Autodesk Inventor part; units mm, degrees
ref_plane "YZ Plane" through (0, 0, 0) normal (1, 0, 0) x (0, 1, 0)
ref_plane "XZ Plane" through (0, 0, 0) normal (0, 1, 0) x (-1, 0, 0)
ref_plane "XY Plane" through (0, 0, 0) normal (0, 0, 1) x (1, 0, 0)
sketch "Sketch1" plane through (0, 0, 0) normal (0, 1, 0) x (-1, 0, 0)
  line L0 (0, 0) -> (60, 0)
  line L1 (60, 0) -> (60, -60)
  line L2 (60, -60) -> (0, -60)
  line L3 (0, -60) -> (0, 0)
  dimension "d0" = 60
  dimension "d1" = 60
extrude "Extrusion1" add sketch "Sketch1" along normal blind 3
sketch "Sketch2" plane through (0, 3, 0) normal (0, 1, 0) x (1, 0, 0)
  line L0 (-60, 0) -> (0, 0)
  line L1 (-60, 60) -> (-60, 0)
  point P0 (-55, 5)
  dimension "d4" = 5
  dimension "d5" = 5
hole "Hole1" at (-55, 3, -5) direction (0, -1, 0) diameter 3 end through all
ref_plane "Work Plane1" through (-30, 0, -60) normal (-1, 0, 0) x (0, 0, 1)
ref_plane "Work Plane2" through (-60, 0, -30) normal (0, 0, 1) x (1, 0, 0)
mirror "Mirror1" about plane through (-30, 0, -60) normal (-1, 0, 0) of "Hole1"
mirror "Mirror2" about plane through (-60, 0, -30) normal (0, 0, 1) of "Hole1", "Mirror1"
sketch "Sketch3" plane through (0, 0, 0) normal (0, -1, 0) x (1, 0, 0)
  line L0 (-39.5, 0) -> (-34.5, 0)
  line L1 (-34.5, 0) -> (-34.5, -60)
  line L2 (-34.5, -60) -> (-39.5, -60)
  line L3 (-39.5, -60) -> (-39.5, 0)
  line L4 (0, -60) -> (-60, -60)
  line L5 (-60, 0) -> (0, 0)
  line L6 (-30, -72) -> (-30, 12)
  dimension "d13" = 5
  dimension "d14" = 4.5
extrude "Extrusion2" add sketch "Sketch3" along normal blind 10 contours L0 L1 L2 L3
sketch "Sketch4" plane through (-34.5, 0, 0) normal (1, 0, 0) x (0, 0, -1)
  line L0 (0, 0) -> (0, -10)
  line L1 (60, 0) -> (60, -10)
  line L2 (0, 0) -> (60, 0)
  line L3 (60, -10) -> (0, -10)
  point P0 (5, -7)
  point P1 (55, -7)
  dimension "d17" = 5
  dimension "d18" = 5
  dimension "d20" = 3
  dimension "d21" = 3
hole "Hole2" at (-34.5, -7, -5) at (-34.5, -7, -55) direction (-1, 0, 0) diameter 3 end through all
mirror "Mirror3" about plane through (-30, 0, -60) normal (-1, 0, 0) of "Extrusion2", "Hole2"
properties part number "Slege_Mounting_Plate"
Read the model definition and answer for the solid it produces. Units are mm, in the model's axes. A direction names the side the tool comes from. Coordinates: 2 decimals unless noted, no trailing zeros. Order: outer loops, then holes, each group sorted by start corner. A loop starts at its lowest first (then second) coordinate and runs counter-clockwise, first axis right, second up. Notation, with made-up numbers: (89.5, 29.25) - (122.5, 29.25) arc R10 cw to (122.5, 33.25) - close; hole circle Ø3 at (78, 34). An arc over 180 degrees is marked (long way). Answer as a JSON object with one key per item and string values. Group by question number.
Item 1: Section C-C (y = -0.75) is taken. Give the vertices of the cut face in (x, z).
Item 2: Section D-D (z = -55) is taken. Give the vertices of the cut face in (x, y).
Item 3: Consider probe 1 along Z at (x, y) = (-35.7, -7); probe 2 along X at (y, z) = (-8.5, -52). Determine where each line is inside the solid, lowest interval first. Write a range as from..to.
Item 4: Flat-ended cylindrical pins translate along their axes: P1, Ø6, axis at x = -55, z = -41, coming from the -Y side; P2, Ø3.5, axis at y = -7, z = -55, coming from the +X side; P3, Ø3, axis at y = -2.5, z = -37.5, coming from the -X side. Find the tip coordinate at first contact, or state that the pin passes through.
Item 5: Section A-A (y = -7) is taken. Give the vertices of the cut face in (x, z), plus the area to 3 significant figures.
Item 6: A tool of negligible diameter and unlimited length cuts with its end or side. For faces 4 (the face through (-30, 0, -30)), 5 (the face through (-50, 0, -30)), 6 (the face through (-54.1, 1.5, -6.2)), 7 (the face through (-10, 0, -30)), from which of +Z, -Z, +X, -X, +Y, -Y can it reach the whole face along a straight path? Write none if from no direction.
Item 7: The mould has two halves that part along X. Classify faces 1 (the face through (-23, -10, -30)), 2 (the face through (-4.1, 1.5, -6.2)), 3 (the face through (-20.5, -5, -30)): +X half, -X half, draft (parallel to the pull), parting line (faces both ways), or undercut.
Item 8: Section B-B (x = -55) is taken. Give the vertices of the cut face in (y, z).
Results are:
{
 "1": {"outline": "(-39.5, -60) - (-34.5, -60) - (-34.5, 0) - (-39.5, 0) - close; (-25.5, -60) - (-20.5, -60) - (-20.5, 0) - (-25.5, 0) - close"},
 "2": {"outline": "(-60, 0) - (-56.5, 0) - (-56.5, 3) - (-60, 3) - close; (-53.5, 0) - (-39.5, 0) - (-39.5, -5.5) - (-34.5, -5.5) - (-34.5, 0) - (-25.5, 0) - (-25.5, -5.5) - (-20.5, -5.5) - (-20.5, 0) - (-6.5, 0) - (-6.5, 3) - (-53.5, 3) - close; (-39.5, -10) - (-34.5, -10) - (-34.5, -8.5) - (-39.5, -8.5) - close; (-25.5, -10) - (-20.5, -10) - (-20.5, -8.5) - (-25.5, -8.5) - close; (-3.5, 0) - (0, 0) - (0, 3) - (-3.5, 3) - close"},
 "3": {"probe 1": "z = -60..-56.5, -53.5..-6.5, -3.5..0", "probe 2": "x = -39.5..-34.5, -25.5..-20.5"},
 "4": {"P1": "stops at y = 0", "P2": "stops at x = -20.5", "P3": "stops at x = -39.5"},
 "5": {"outline": "(-39.5, -60) - (-34.5, -60) - (-34.5, -56.5) - (-39.5, -56.5) - close; (-39.5, -53.5) - (-34.5, -53.5) - (-34.5, -6.5) - (-39.5, -6.5) - close; (-39.5, -3.5) - (-34.5, -3.5) - (-34.5, 0) - (-39.5, 0) - close; (-25.5, -60) - (-20.5, -60) - (-20.5, -56.5) - (-25.5, -56.5) - close; (-25.5, -53.5) - (-20.5, -53.5) - (-20.5, -6.5) - (-25.5, -6.5) - close; (-25.5, -3.5) - (-20.5, -3.5) - (-20.5, 0) - (-25.5, 0) - close", "area": "540 mm^2"},
 "6": {"face 4": "+Z, -Z, -Y", "face 5": "+Z, -Z, -X, -Y", "face 6": "+Y, -Y", "face 7": "+Z, -Z, +X, -Y"},
 "7": {"face 1": "draft", "face 2": "undercut", "face 3": "+X half"},
 "8": {"outline": "(0, -60) - (3, -60) - (3, -56.5) - (0, -56.5) - close; (0, -53.5) - (3, -53.5) - (3, -6.5) - (0, -6.5) - close; (0, -3.5) - (3, -3.5) - (3, 0) - (0, 0) - close"}
}
